```python
from build123d import *

# Parameters (mm, degrees)
SKETCH_1_W          = 20
SKETCH_1_H          = 15
SKETCH_1_R          = 5
EXTRUDE_1_DEPTH     = 40
SKETCH_2_R          = 4
CUT_EXTRUDE_1_DEPTH = 3
SKETCH_3_R          = 2
CUT_EXTRUDE_2_DEPTH = 45.10498838
SKETCH_4_W          = 26.593745906
SKETCH_4_H          = 18.404579196
CUT_EXTRUDE_3_DEPTH = 13
SKETCH_5_R          = 3.5
CUT_EXTRUDE_4_DEPTH = 0.5
CUT_EXTRUDE_5_DEPTH = 6


with BuildPart() as part:
    # 草圖1 → 填料-伸長1 (new body)
    with BuildSketch(Plane(origin=(0, 0, 0), x_dir=(0, 0, -1), z_dir=(1, 0, 0))):
        Rectangle(SKETCH_1_W, SKETCH_1_H)
        Circle(SKETCH_1_R, mode=Mode.SUBTRACT)
    extrude(amount=EXTRUDE_1_DEPTH)

    # 草圖2 → 除料-伸長1 (cut)
    with BuildSketch(Plane.XY.offset(10)):
        with Locations((20, 0)):
            Circle(SKETCH_2_R)
    cut_extrude_1 = extrude(amount=-CUT_EXTRUDE_1_DEPTH, mode=Mode.SUBTRACT)

    # 鏡射1: 除料-伸長1 across plane
    add(cut_extrude_1.mirror(Plane.XY), mode=Mode.SUBTRACT)

    # 草圖3 → 除料-伸長2 (cut, through all)
    with BuildSketch(Plane.XY.offset(7)):
        with Locations(Location((20, 0, 0), (0, 0, 179.999999998))):
            Circle(SKETCH_3_R)
    extrude(amount=-CUT_EXTRUDE_2_DEPTH, mode=Mode.SUBTRACT)

    # 草圖4 → 除料-伸長3 (cut)
    with BuildSketch(Plane.ZY):
        Rectangle(SKETCH_4_W, SKETCH_4_H)
        with BuildLine():
            Line((-6, 7.5), (6, 7.5))
            ThreePointArc((6, 7.5), (8.828427125, 6.328427125), (10, 3.5))
            Line((10, 3.5), (10, -7.5))
            Line((10, -7.5), (-6, -7.5))
            ThreePointArc((-6, -7.5), (-8.828427125, -6.328427125), (-10, -3.5))
            Line((-10, -3.5), (-10, 3.5))
            ThreePointArc((-10, 3.5), (-8.828427125, 6.328427125), (-6, 7.5))
        make_face(mode=Mode.SUBTRACT)
    cut_extrude_3 = extrude(amount=-CUT_EXTRUDE_3_DEPTH, mode=Mode.SUBTRACT)

    # 鏡射2: 除料-伸長3 across plane
    add(cut_extrude_3.mirror(Plane(origin=(20, 0, 0), x_dir=(0, 0, 1), z_dir=(1, 0, 0))), mode=Mode.SUBTRACT)

    # 草圖5 → 除料-伸長4 (cut)
    with BuildSketch(Plane(origin=(0, 0, -7), x_dir=(-1, 0, 0), z_dir=(0, 0, -1))):
        with Locations((-20, 0)):
            Circle(SKETCH_5_R)
    cut_extrude_4 = extrude(amount=-CUT_EXTRUDE_4_DEPTH, mode=Mode.SUBTRACT)

    # 鏡射3: 除料-伸長4 across plane
    add(cut_extrude_4.mirror(Plane.XY), mode=Mode.SUBTRACT)

    # 草圖6 → 除料-伸長5 (cut)
    with BuildSketch(Plane.XY.offset(-10)):
        with BuildLine():
            Line((15.669872981, -7.5), (24.330127019, -7.5))
            Line((24.330127019, -7.5), (33.279056191, -7.5))
            Line((33.279056191, -7.5), (30.418218618, -2.544883972))
            Line((30.418218618, -2.544883972), (27.729646072, -1.888139721))
            Line((27.729646072, -1.888139721), (22.75, -4.763139721))
            ThreePointArc((22.75, -4.763139721), (20, -5.5), (17.25, -4.763139721))
            Line((17.25, -4.763139721), (12.270353928, -1.888139721))
            Line((12.270353928, -1.888139721), (9.581781382, -2.544883972))
            Line((9.581781382, -2.544883972), (6.720943809, -7.5))
            Line((6.720943809, -7.5), (15.669872981, -7.5))
        make_face()
    extrude(amount=CUT_EXTRUDE_5_DEPTH, mode=Mode.SUBTRACT)


solid = part.part
```
The model under review builds one solid part; all positions refer to its coordinate system, in mm. A direction names the side the tool comes from. Round coordinates to 2 decimals unless told otherwise and drop trailing zeros. Order: outer loops, then holes, each group sorted by start corner. A loop starts at its lowest first (then second) coordinate and runs counter-clockwise, first axis right, second up.
Item 1: Add section D-D, the plane y = 2.5. State the section outline as (x, z) points.
Working result:
outline: (0, -10) - (16.88, -10) - (16.88, -7) - (17.55, -7) - (17.55, -6.5) - (22.45, -6.5) - (22.45, -7) - (23.12, -7) - (23.12, -10) - (40, -10) - (40, -4.33) - (0, -4.33) - close; (0, 4.33) - (40, 4.33) - (40, 10) - (23.12, 10) - (23.12, 7) - (22.45, 7) - (22.45, 6.5) - (17.55, 6.5) - (17.55, 7) - (16.88, 7) - (16.88, 10) - (0, 10) - close
Item 2: Machinability: for faces 1 (the cylindrical face through (16.8, -2.4, -8.5)), 2 (the flat face through (31.87, -5.06, -7.04)), 3 (the cylindrical face through (3.449, -6.359, -8.797)), 4 (the cylindrical face through (16.8, -2.4, 8.5)), which of the approach directions +Z, -Z, +X, -X, +Y, -Y give a long, thin tool a straight path to every point of the face, cutting with its end or side? Answer none if there is none.
Working result:
face 1: -Z
face 2: -Z, -Y
face 3: -Z, -X, -Y
face 4: +Z
Item 3: For pin 1 (2 mm diameter, centred on x = 19, y = 1, fed in from -Z); pin 2 (5 mm diameter, centred on x = 20, y = 0, fed in from +Z); pin 3 (3 mm diameter, centred on x = 11.5, z = -6.5, fed in from -Y), all flat-tipped, find the tip position at first contact; note any pin that passes through.
Working result:
pin 1: stops at z = -6.5
pin 2: stops at z = 6.5
pin 3: stops at y = -2.44
Item 4: Add section A-A, the plane y = 0. Count the separate pieces of the cut face and the enclosed holes in it, and give its area (3 significant figures).
Working result:
separate pieces: 4
enclosed holes: 0
area: 333 mm2
Item 5: Draft analysis for pull direction X (two halves, no side actions). For faces 5 (the cylindrical face through (20, -5.5, -7)), 6 (the flat face through (20, 7.5, 0)), 7 (the flat face through (13, 7, 9)), state which applies: released by +X, released by -X, zero draft, split by the parting line, or undercut.
Working result:
face 5: undercut
face 6: zero draft
face 7: released by -X
Item 6: Add section C-C, the plane z = 0. State the section outline as (x, y) points, and give its area (3 significant figures).
Working result:
outline: (0, -7.5) - (40, -7.5) - (40, -5) - (0, -5) - close; (0, 5) - (40, 5) - (40, 7.5) - (0, 7.5) - close
area: 200 mm2
Item 7: To check wall thickness, follow probe 1 along Z at (x, y) = (38, 3); probe 2 along Y at (x, z) = (20, -6.6); probe 3 along Y at (x, z) = (20, 9.2). State the ranges of each line that lie inside material, in increasing order.
Working result:
probe 1: z = -10 to -4, 4 to 10
probe 2: y = -5.5 to -3.5, 3.5 to 7.5
probe 3: y = -7.5 to -4, 4 to 7.5
